Can you work these out from the model? Positions are in its coordinate system, mm. Face numbers are marked on the shaded views. A direction names the side the tool comes from. Round coordinates to 2 decimals unless told otherwise and drop trailing zeros. Loops run counter-clockwise (first coordinate to the right, second up) from the corner with the lowest first, then second, coordinate; pieces in that order, holes last.
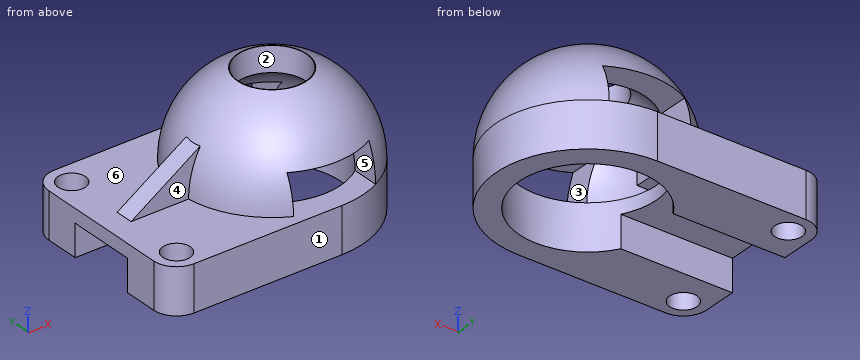
Autodesk Fusion 360 part; units mm, degrees
sketch "Sketch1" plane through (0, 0, 0) normal (0, 0, 1) x (1, 0, 0)
  line L0 (0, 0) -> (37.5, 0)
  line L1 (0, 0) -> (-37.5, 0)
  line L2 (-37.5, 0) -> (-37.5, 40)
  line L3 (37.5, 0) -> (37.5, -40)
  line L4 (-37.5, 40) -> (37.5, 40)
  line L5 (37.5, 40) -> (37.5, -40)
  line L6 (37.5, -40) -> (-37.5, -40)
  line L7 (-37.5, -40) -> (-37.5, 40)
  dimension "d1" = 37.5
  dimension "d2" = 37.5
  dimension "d3" = 40
  dimension "d4" = 40
extrude "Extrude1" add sketch "Sketch1" along normal blind 20 makes body 1
sketch "Sketch2" plane through (0, 0, 20) normal (0, 0, 1) x (-1, 0, 0)
  line L0 (37.5, 40) -> (-37.5, 40)
  line L1 (-37.5, 40) -> (-37.5, -40)
  line L2 (-37.5, -40) -> (37.5, -40)
  line L3 (37.5, -40) -> (37.5, 40)
  line L4 (37.5, 0) -> (37.5, -30)
  line L5 (37.5, 0) -> (37.5, 30)
  line L6 (-37.5, -40) -> (27.5, -40)
  circle A0 centre (27.5, -30) radius 6
  circle A1 centre (27.5, 30) radius 6
  point P0 (37.5, 0)
  dimension "d8" = 30
  dimension "d10" = 12
  dimension "d11" = 12
extrude "Extrude2" cut sketch "Sketch2" against normal blind 90 contours A0 | A1 bodies 1
sketch "Sketch3" plane through (0, 0, 20) normal (0, 0, 1) x (-1, 0, 0)
  circle A0 centre (27.5, 30) radius 6
  circle A1 centre (27.5, -30) radius 6
  line L0 (37.5, 40) -> (-37.5, 40)
  line L1 (-37.5, 40) -> (-37.5, -40)
  line L2 (-37.5, -40) -> (37.5, -40)
  line L3 (37.5, -40) -> (37.5, 40)
  circle A2 centre (27.5, 30) radius 10
  circle A3 centre (27.5, -30) radius 10
  dimension "d14" = 20
  dimension "d15" = 20
extrude "Extrude3" cut sketch "Sketch3" against normal blind 35 contours L0 L3 A2 | L2 L3 A3 bodies 1
sketch "Sketch4" plane through (0, 0, 20) normal (0, 0, 1) x (-1, 0, 0)
  arc A0 (37.5, 30) -> (27.5, 40) centre (27.5, 30) ccw
  line L0 (27.5, 40) -> (-37.5, 40)
  line L1 (-37.5, 40) -> (-37.5, -40)
  line L2 (-37.5, -40) -> (27.5, -40)
  arc A1 (27.5, -40) -> (37.5, -30) centre (27.5, -30) ccw
  line L3 (37.5, -30) -> (37.5, 30)
  circle A2 centre (27.5, 30) radius 6
  circle A3 centre (27.5, -30) radius 6
  circle A4 centre (-37.5, 0) radius 40
  dimension "d18" = 80
extrude "Extrude4" add sketch "Sketch4" against normal blind 20 contours L1 A4 | L1 A4 bodies 1
sketch "Sketch5" plane through (0, 0, 0) normal (0, 0, -1) x (1, 0, 0)
  line L0 (37.5, 40) -> (-27.5, 40)
  arc A0 (-27.5, 40) -> (-37.5, 30) centre (-27.5, 30) ccw
  line L1 (-37.5, 30) -> (-37.5, -30)
  arc A1 (-37.5, -30) -> (-27.5, -40) centre (-27.5, -30) ccw
  line L2 (-27.5, -40) -> (37.5, -40)
  arc A2 (37.5, -40) -> (37.5, 40) centre (37.5, 0) ccw
  circle A3 centre (-27.5, 30) radius 6
  circle A4 centre (-27.5, -30) radius 6
  point P0 (37.5, 0)
sphere "SpherePrimitive1" add diameter 80 placed x (-1, 0, 0) y (0, -1, 0) z (0, 0, 1) at (37.5, 0, 20) bodies 1
extrude "Extrude5" cut sketch "Sketch5" along normal blind 20 bodies 1
sketch "Sketch7" plane through (0, 0, 0) normal (0, 0, -1) x (1, 0, 0)
  line L0 (37.5, 40) -> (-27.5, 40)
  arc A0 (-27.5, 40) -> (-37.5, 30) centre (-27.5, 30) ccw
  line L1 (-37.5, 30) -> (-37.5, -30)
  arc A1 (-37.5, -30) -> (-27.5, -40) centre (-27.5, -30) ccw
  line L2 (-27.5, -40) -> (37.5, -40)
  arc A2 (37.5, -40) -> (37.5, 40) centre (37.5, 0) ccw
  circle A3 centre (-27.5, 30) radius 6
  circle A4 centre (-27.5, -30) radius 6
  circle A5 centre (37.5, 0) radius 30
  dimension "d24" = 60
extrude "Extrude6" cut sketch "Sketch7" against normal blind 20 contours A5 bodies 1
sphere "SpherePrimitive2" cut diameter 60 placed x (1, 0, 0) y (0, -1, 0) z (0, 0, -1) at (37.5, 0, 20) bodies 1
sketch "Sketch9" plane through (0, 0, 0) normal (0, 0, 1) x (1, 0, 0)
ref_plane "WorkPlane1" through (0, 0, 57) normal (0, 0, 1) x (1, 0, 0)
sketch "Sketch10" plane through (0, 0, 57) normal (0, 0, 1) x (1, 0, 0)
  line L0 (7.4967, 46.768) -> (98.4073, 46.768)
  line L1 (98.4073, 46.768) -> (98.4073, -40.4525)
  line L2 (98.4073, -40.4525) -> (7.4967, -40.4525)
  line L3 (7.4967, -40.4525) -> (7.4967, 46.768)
extrude "Extrude7" cut sketch "Sketch10" along normal blind 20 bodies 1
sketch "Sketch11" plane through (0, 0, 57) normal (0, 0, 1) x (-1, 0, 0)
  circle A0 centre (-37.5, 0) radius 15.1987
  circle A1 centre (-37.5, 0) radius 15
  dimension "d31" = 30
extrude "Extrude8" cut sketch "Sketch11" against normal blind 15 contours A1 bodies 1
sketch "Sketch12" plane through (0, 0, 20) normal (0, 0, 1) x (-1, 0, 0)
  arc A0 (-37.5, -40) -> (-37.5, 40) centre (-37.5, 0) ccw
  line L0 (-37.5, -40) -> (27.5, -40)
  arc A1 (27.5, -40) -> (37.5, -30) centre (27.5, -30) ccw
  line L1 (37.5, -30) -> (37.5, 30)
  arc A2 (37.5, 30) -> (27.5, 40) centre (27.5, 30) ccw
  line L2 (27.5, 40) -> (-37.5, 40)
  circle A3 centre (27.5, 30) radius 6
  circle A4 centre (27.5, -30) radius 6
  line L3 (-37.5, 40) -> (27.5, 40)
  line L4 (27.5, 0) -> (27.5, -4)
  line L5 (27.5, -4) -> (27.5, 0)
  line L6 (27.5, 0) -> (27.5, 4)
  line L7 (27.5, 4) -> (0, 4)
  line L8 (0, 4) -> (0, -4)
  line L9 (0, -4) -> (27.5, -4)
  line L10 (27.5, -4) -> (0, -4)
  line L11 (0, -4) -> (0, 4)
  line L12 (0, 4) -> (27.5, 4)
  line L13 (27.5, 4) -> (27.5, -4)
  line L14 (27.5, -4) -> (-12.731, -4)
  line L15 (-12.731, -4) -> (-12.731, 4)
  line L16 (-12.731, 4) -> (27.5, 4)
  line L17 (27.5, 4) -> (27.5, -4)
  point P0 (37.5, 0)
  dimension "d34" = 65
  dimension "d37" = 8
extrude "Extrude9" add sketch "Sketch12" along normal blind 26 separate body contours A0 L7 L8 L9 L10 L11 L12 L14 L16 | A0 L4 L5 L6 L7 L9 L10 L12 L13 L14 L16 L17 | L8 L11 L14 L15 L16 makes body 2
sketch "Sketch13" plane through (0, 4, 0) normal (0, 1, 0) x (-1, 0, 0)
  line L0 (-12.731, 20) -> (27.5, 20)
  line L1 (27.5, 20) -> (27.5, 46)
  line L2 (27.5, 46) -> (-12.731, 46)
  line L3 (-12.731, 46) -> (-12.731, 20)
  line L4 (-12.731, 46) -> (27.5, 20)
extrude "Extrude10" cut sketch "Sketch13" against normal blind 24 contours L1 L2 L4 bodies 2
combine "Combine1" operation add target body 2 tool bodies 1
sketch "Sketch14" plane through (-37.5, 0, 0) normal (-1, 0, 0) x (0, -1, 0)
  line L0 (30, 0) -> (30, 20)
  line L1 (30, 20) -> (-30, 20)
  line L2 (-30, 20) -> (-30, 0)
  line L3 (-30, 0) -> (30, 0)
  line L4 (0, 0) -> (-15, 0)
  line L5 (0, 0) -> (15, 0)
  line L6 (-15, 0) -> (15, 0)
  line L7 (15, 0) -> (15, 14)
  line L8 (15, 14) -> (-15, 14)
  line L9 (-15, 14) -> (-15, 0)
  dimension "d42" = 15
  dimension "d44" = 14
extrude "Extrude11" cut sketch "Sketch14" against normal blind 75 contours L3 L4 L5 L6 L7 L8 L9 bodies 2
sketch "Sketch15" plane through (0, -40, 0) normal (0, -1, 0) x (1, 0, 0)
  line L0 (-27.5, 20) -> (-27.5, 0)
  line L1 (-27.5, 0) -> (37.5, 0)
  line L2 (37.5, 20) -> (-27.5, 20)
  line L3 (37.5, 20) -> (37.5, 36)
  line L4 (37.5, 36) -> (55.5, 36)
  line L5 (55.5, 36) -> (37.5, 36)
  line L6 (37.5, 36) -> (19.5, 36)
  line L7 (55.5, 36) -> (55.5, 20)
  line L8 (19.5, 36) -> (55.5, 36)
  line L9 (55.5, 36) -> (55.5, 20)
  line L10 (55.5, 20) -> (19.5, 20)
  line L11 (19.5, 20) -> (19.5, 36)
  dimension "d47" = 16
  dimension "d48" = 18
  dimension "d49" = 18
extrude "Extrude12" cut sketch "Sketch15" against normal blind 105 bodies 2
(1) If I drill on line 1 (Y direction, x = 8.5, z = 11); line 2 (Y direction, x = -27, z = 15); line 3 (Y direction, x = 37.5, z = 13.5), over which ranges is the centre line in solid material (lowest first)?
Worked answers:
line 1: y = -40 to -15, 15 to 40
line 2: y = -40 to -35.98, -24.02 to 24.02, 35.98 to 40
line 3: y = -40 to -30, 30 to 40
(2) If we section it at A-A, the plane x = -23.5: List the corners of the cut face in (y, z) for me, then the cut area to 3 significant figures.
Worked answers:
outline: (-40, 0) - (-34.47, 0) - (-34.47, 20) - (-40, 20) - close; (-25.53, 0) - (-15, 0) - (-15, 14) - (15, 14) - (15, 0) - (25.53, 0) - (25.53, 20) - (4, 20) - (4, 22.59) - (-4, 22.59) - (-4, 20) - (-25.53, 20) - close; (34.47, 0) - (40, 0) - (40, 20) - (34.47, 20) - close
area: 843 mm2
(3) If we section it at D-D, the plane z = 23.5: List the corners of the cut face in (x, y) for me.
Worked answers:
outline: (-22.08, -4) - (-2.15, -4) arc R39.85 ccw to (19.5, -35.55) - (19.5, -23.74) arc R29.8 cw to (7.97, -4) - (12.73, -4) - (12.73, 4) - (7.97, 4) arc R29.8 cw to (19.5, 23.74) - (19.5, 35.55) arc R39.85 ccw to (-2.15, 4) - (-22.08, 4) - close; (55.5, -35.55) arc R39.85 ccw to (55.5, 35.55) - (55.5, 23.74) arc R29.8 cw to (55.5, -23.74) - close
(4) Will these pins go through, and if not, where does the flat tip stop? P1, Ø2, axis at x = -6.5, y = -9, coming from the -Z side; P2, Ø5, axis at y = 29.5, z = 35.5, coming from the -X side; P3, Ø12, axis at y = -18, z = 35.5, coming from the -X side.
Worked answers:
P1: stops at z = 14
P2: stops at x = 12.01
P3: stops at x = 1.66
(5) If we section it at C-C, the plane y = -8: List the corners of the cut face in (x, z) for me.
Worked answers:
outline: (-37.5, 14) - (8.59, 14) - (8.59, 20) arc R28.91 cw to (24.81, 45.98) - (24.81, 57) - (24.58, 57) arc R39.19 ccw to (-1.69, 20) - (-37.5, 20) - close; (50.19, 45.98) arc R28.91 cw to (66.41, 20) - (66.41, 0) - (76.69, 0) - (76.69, 20) arc R39.19 ccw to (50.42, 57) - (50.19, 57) - close
(6) If we section it at B-B, the plane z = 15.5: List the corners of the cut face in (x, y) for me.
Worked answers:
outline: (-37.5, -30) arc R10 ccw to (-27.5, -40) - (37.5, -40) arc R40 ccw to (37.5, 40) - (-27.5, 40) arc R10 ccw to (-37.5, 30) - close; hole circle Ø12 at (-27.5, -30); hole circle Ø12 at (-27.5, 30); hole circle Ø60 at (37.5, 0)
(7) For the marked faces 4, 5 and 6, which set-ups out of +Z, -Z, +X, -X, +Y, -Y let a thin tool reach every point of the face, with its end or its side?
Worked answers:
face 4: +Z, -X, -Y
face 5: +Y, -Y
face 6: none
(8) If we mould it in two halves opening along Y, with no side actions, what happens to the marked faces 1, 2 and 3? For each: released by +Y, released by -Y, zero draft, split by the parting line, or undercut.
Worked answers:
face 1: released by -Y
face 2: undercut
face 3: zero draft
